```python
from build123d import *

# Parameters (mm, degrees)
CHAMFER1_SIZE = 0.127


with BuildPart() as part:
    # Sketch1 → Revolve1 (revolve)
    with BuildSketch(Plane.XY, mode=Mode.PRIVATE) as revolve1_sk:
        with BuildLine():
            Line((-8.7122, 0.381), (-8.7122, 1.143))
            Line((-8.7122, 1.143), (-7.9375, 1.143))
            Line((-7.9375, 1.143), (-7.9375, 4.318))
            Line((-7.9375, 4.318), (-7.636387191, 10.063574666))
            ThreePointArc((-7.636387191, 10.063574666), (-7.063125107, 10.61711204), (-6.471000704, 10.0838))
            Line((-6.471000704, 10.0838), (-6.0198, 10.0838))
            Line((-6.0198, 10.0838), (-6.0198, 10.795))
            Line((-6.0198, 10.795), (-5, 10.795))
            Line((-5, 10.795), (-5, 0))
            Line((-5, 0), (-6.0198, 0))
            Line((-6.0198, 0), (-6.0198, 1.651))
            Line((-6.0198, 1.651), (-6.4008, 1.651))
            Line((-6.4008, 1.651), (-6.4008, 0.381))
            Line((-6.4008, 0.381), (-8.7122, 0.381))
        make_face()
    revolve(revolve1_sk.sketch.rotate(Axis((0, 15.281488856, 0), (0, -1, 0)), 270), axis=Axis((0, 15.281488856, 0), (0, -1, 0)))

    # Chamfer1
    chamfer1_edges = [part.edges().sort_by_distance(p)[0] for p in [
        (0, 0, -6.0198),
        (0, 0, -5),
        (0, 10.795, -5),
        (0, 10.795, -6.0198),
        (0, 0.381, -6.4008),
    ]]
    chamfer(chamfer1_edges, length=CHAMFER1_SIZE)


solid = part.part
```
Work out the finished part from the listing and answer in its coordinate system (mm). A direction names the side the tool comes from. Give positions to 0.01 mm unless a question says otherwise; leave off trailing zeros. Write each loop counter-clockwise with the first axis right and the second up, starting at its lowest first coordinate (ties: lowest second). Pieces come first, ordered by that corner, then holes.
(1) The part is cut by section A-A on y = 3.75. Write down the section's boundary in (x, z) (1 decimal).
Final values:
outline: circle Ø15.9 at (0, 0); hole circle Ø10 at (0, 0)
(2) The mould has two halves that part along X. Classify faces 1 (the cylindrical face through (4.88, 5.32, -1.08)), 2 (the cylindrical face through (-1.81, 0.9, 5.74)), 3 (the flat face through (3.5, 0, 4)), 4 (the cylindrical face through (7.75, 2.75, -1.72)): pulls with the +X half, pulls with the -X half, needs draft (parallel to the pull), parting line crosses it, or undercut.
Final values:
face 1: undercut
face 2: undercut
face 3: needs draft
face 4: parting line crosses it
(3) Flat-ended cylindrical pins translate along their axes: pin 1 Ø2 at (x, y) = (6.5, 6.5) entering from -Z; pin 2 Ø1 at (y, z) = (2, -4.5) entering from -X; pin 3 Ø8.5 at (x, z) = (2.5, 4) entering from -Y; pin 4 Ø3 at (y, z) = (5.5, -2) entering from -X. Find the tip coordinate at first contact, or state that the pin passes through.
Final values:
pin 1: stops at z = -5.57
pin 2: stops at x = -6.86
pin 3: stops at y = 0
pin 4: stops at x = -7.88
(4) The part is cut by section B-B on y = 5. Write down the section's boundary in (x, z), plus the area to 3 significant figures.
Final values:
outline: circle Ø15.8 at (0, 0); hole circle Ø10 at (0, 0)
area: 118 mm2
(5) Which of the six approach directions +Z, -Z, +X, -X, +Y, -Y give full straight-line access (tool end or side, diameter ignored) to faces 5 (the cylindrical face through (3.895, 1.071, -5.079)), 6 (the cylindrical face through (-2.62, 0.77, 8.31)), 7 (the flat face through (-2, 1.143, 8))?
Final values:
face 5: -Y
face 6: +Y, -Y
face 7: +Y
(6) Straight lines are drawn through the part: line 1 (X direction, y = 0.85, z = 0); line 2 (X direction, y = 3.75, z = 0); line 3 (X direction, y = 1.5, z = 3.75). For each, find the intervals that lie inside material, in ascending order.
Final values:
line 1: x = -8.71 to -6.4, -6.02 to -5, 5 to 6.02, 6.4 to 8.71
line 2: x = -7.94 to -5, 5 to 7.94
line 3: x = -7 to -5.19, -4.71 to -3.31, 3.31 to 4.71, 5.19 to 7
